Verification items for the finished model (mm, model axes). A direction names the side the tool comes from. Coordinates: 2 decimals unless noted, no trailing zeros. Order: outer loops, then holes, each group sorted by start corner. A loop starts at its lowest first (then second) coordinate and runs counter-clockwise, first axis right, second up. Notation, with made-up numbers: M -25.5,-5.75 L 11.5,-5.75 A23 cw 11.5,32.25 Z; hole C -29,10.5 d3. An arc over 180 degrees is marked long. Return JSON: item names as keys, results as strings.
```python
from build123d import *

# Parameters (mm, degrees)
SKETCH_1_R        = 0.3
EXTRUDE_5_DEPTH   = 7
EXTRUDE_5_2_DEPTH = 7
EXTRUDE_5_3_DEPTH = 7
EXTRUDE_6_DEPTH   = 0.5
SKETCH_6_R        = 2.45
EXTRUDE_7_DEPTH   = 8.5
CHAMFER_1_SIZE    = 0.5


with BuildPart() as part:
    # Sketch 1 → Extrude 5 (new body)
    with BuildSketch(Plane.XY):
        with Locations((-1.27, 1.05)):
            Circle(SKETCH_1_R)
    extrude(amount=EXTRUDE_5_DEPTH)



with BuildPart() as body_2:
    # Sketch 1 → Extrude 5 2 (new body)
    with BuildSketch(Plane.XY):
        with Locations((1.27, 1.05)):
            Circle(SKETCH_1_R)
    extrude(amount=EXTRUDE_5_2_DEPTH)


with BuildPart() as body_3:
    # Sketch 1 → Extrude 5 3 (new body)
    with BuildSketch(Plane.XY):
        with Locations((0, -1.05)):
            Circle(SKETCH_1_R)
    extrude(amount=EXTRUDE_5_3_DEPTH)


with BuildPart() as part_1:
    add(part.part)

    add(body_2.part)  # Extrude 6 merges body 2

    add(body_3.part)  # Extrude 6 merges body 3
    # Sketch 5 → Extrude 6 (add)
    with BuildSketch(Plane.XY.offset(7)):
        with BuildLine():
            Line((-1.34079253, 2.400994667), (1.34079253, 2.400994667))
            ThreePointArc((1.34079253, 2.400994667), (0, -2.75), (-1.34079253, 2.400994667))
        make_face()
    extrude(amount=EXTRUDE_6_DEPTH)

    # Sketch 6 → Extrude 7 (add)
    with BuildSketch(Plane.XY.offset(7.5)):
        with Locations(Location((0, 0, 0), (0, 0, 101.478967652))):
            Circle(SKETCH_6_R)
    extrude(amount=EXTRUDE_7_DEPTH)

    # Chamfer 1
    chamfer_1_edges = [part_1.edges().sort_by_distance(p)[0] for p in [
        (0.487570106, -2.400994667, 16),
    ]]
    chamfer(chamfer_1_edges, length=CHAMFER_1_SIZE)


solid = part_1.part
```
Q1. Material ranges on line 1 along Z through (x, y) = (-0.95, 1.2); line 2 along Z through (x, y) = (0.8, -2.5); line 3 along Y through (x, z) = (1.2, 5), recorded low to high.
Values:
{"line 1": "7 to 16", "line 2": "7 to 7.5", "line 3": "0.76 to 1.34"}
Q2. Cross-section at D-D, the plane z = 13.5. Record the boundary of the cut face in (x, y).
Values:
{"outline": "C 0,0 d4.9"}
Q3. Go/stop test with flat-tipped pins: pin 1 (1.5 mm diameter, centred on x = -1, y = -1, fed in from -Z); pin 2 (1.5 mm diameter, centred on y = 0, z = 11, fed in from -X); pin 3 (1 mm diameter, centred on y = -0.5, z = 3, fed in from -X); pin 4 (1 mm diameter, centred on x = -2, y = 0, fed in from -Z). Record where each tip stops, or that it passes through.
Values:
{"pin 1": "z = 0", "pin 2": "x = -2.45", "pin 3": "x = -0.3", "pin 4": "z = 7"}
Q4. Cross-section at C-C, the plane x = 0. Record the boundary of the cut face in (y, z), and give its area (3 significant figures).
Values:
{"outline": "M -2.75,7 L -1.35,7 L -1.35,0 L -0.75,0 L -0.75,7 L 2.4,7 L 2.4,7.5 L 2.45,7.5 L 2.45,15.5 L 1.95,16 L -1.95,16 L -2.45,15.5 L -2.45,7.5 L -2.75,7.5 Z", "area": "48.2 mm^2"}
Q5. Tool access check on faces 1 (the face through (-1.19, 2.14, 11.44)), 2 (the face through (0, 0, 7)), 3 (the face through (0.1, -2.75, 7.25)). Record the directions out of +Z, -Z, +X, -X, +Y, -Y that give a thin tool (end or side, any length) a straight path to the whole face; none if there is none.
Values:
{"face 1": "+Z", "face 2": "-Z", "face 3": "+Z, -Z"}
Q6. Cross-section at B-B, the plane z = 5. Record the boundary of the cut face in (x, y), and give its area (3 significant figures).
Values:
{"outline": "C -1.27,1.05 d0.6; C 0,-1.05 d0.6; C 1.27,1.05 d0.6", "area": "0.848 mm^2"}
Q7. Cross-section at A-A, the plane y = 0. Record the boundary of the cut face in (x, z).
Values:
{"outline": "M -2.75,7 L 2.75,7 L 2.75,7.5 L 2.45,7.5 L 2.45,15.5 L 1.95,16 L -1.95,16 L -2.45,15.5 L -2.45,7.5 L -2.75,7.5 Z"}
